Source: CAD feature listing. Evaluate the final solid. Frame: model axes, mm. Face numbers are marked on the shaded views. A direction names the side the tool comes from. Give positions to 0.01 mm unless a question says otherwise; leave off trailing zeros. Order: outer loops, then holes, each group sorted by start corner. A loop starts at its lowest first (then second) coordinate and runs counter-clockwise, first axis right, second up. Notation, with made-up numbers: (83.25, 89) - (93.25, 89) arc R14 cw to (93.25, 102) - close; hole circle Ø11 at (-10.75, -26.5). An arc over 180 degrees is marked (long way). Use CSV: the item, a comma, the result in double quotes.
```python
from build123d import *

# Parameters (mm, degrees)
CUT_EXTRUDE1_DEPTH      = 113.41663578
CUT_EXTRUDE1_DEPTH_BACK = 113.41663578
SKETCH6_R               = 16.9


with BuildPart() as part:
    # Sketch5 → Revolve1 (revolve)
    with BuildSketch(Plane.XY, mode=Mode.PRIVATE) as revolve1_sk:
        with BuildLine():
            Line((25, 0), (42.5, 0))
            Line((42.5, 0), (42.5, 55.2))
            Line((42.5, 55.2), (39.5, 55.2))
            Line((39.5, 55.2), (39.5, 59.5))
            Line((39.5, 59.5), (42.5, 59.5))
            Line((42.5, 59.5), (42.5, 66.8))
            Line((42.5, 66.8), (39.5, 66.8))
            Line((39.5, 66.8), (39.5, 71.1))
            Line((39.5, 71.1), (42.5, 71.1))
            Line((42.5, 71.1), (42.5, 78.4))
            Line((42.5, 78.4), (39.5, 78.4))
            Line((39.5, 78.4), (39.5, 82.7))
            Line((39.5, 82.7), (42.5, 82.7))
            Line((42.5, 82.7), (42.5, 90))
            ThreePointArc((42.5, 90), (21.396553461, 93.745704417), (0, 95))
            Line((0, 95), (0, 90))
            Line((0, 90), (0, 85))
            Line((0, 85), (38, 85))
            Line((38, 85), (38, 49.5))
            Line((38, 49.5), (19, 49.5))
            Line((19, 49.5), (19, 12))
            Line((19, 12), (25, 12))
            Line((25, 12), (25, 0))
        make_face()
    revolve(revolve1_sk.sketch.rotate(Axis((0, 0, 0), (0, 1, 0)), 90), axis=Axis((0, 0, 0), (0, 1, 0)))

    # Sketch6 → Cut-Extrude1 (cut, two sides: drawn at the far end of the back side and taken through both)
    with BuildSketch(Plane.XY.offset(-CUT_EXTRUDE1_DEPTH_BACK)):
        with Locations((0, 27)):
            Circle(SKETCH6_R)
    extrude(amount=CUT_EXTRUDE1_DEPTH + CUT_EXTRUDE1_DEPTH_BACK, mode=Mode.SUBTRACT)


solid = part.part
```
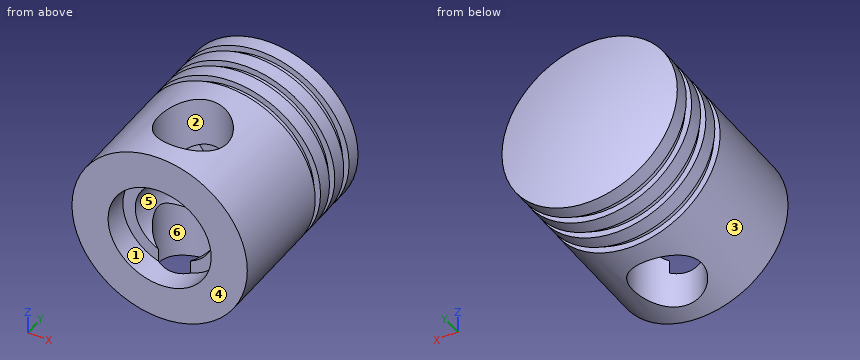
Item 1: Section D-D on y = 73. Return the cut outline in (x, z), then the cut area to 3 significant figures.
Filled in:
outline,"circle Ø85 at (0, 0); hole circle Ø76 at (0, 0)"
area,"1,140 mm2"
Item 2: Material intervals for line 1 (X direction, y = 30, z = 0); line 2 (Y direction, x = 0, z = 31); line 3 (Y direction, x = 6, z = 37), sorted ascending. Write a range as from..to.
Filled in:
line 1,"x = -42.5..-19, 19..42.5"
line 2,"y = 0..10.1, 43.9..49.5, 85..92.36"
line 3,"y = 0..11.2, 42.8..49.5, 85..91.12"
Item 3: First-contact query: pin 1 (5 mm diameter, centred on y = 55, z = 21.5, fed in from +X); pin 2 (14 mm diameter, centred on x = -18.5, z = -9.5, fed in from -Y); pin 3 (6 mm diameter, centred on x = 23, y = 33.5, fed in from +Z); pin 4 (6 mm diameter, centred on y = 58.5, z = 32, fed in from -X). Flat tips, straight axial feed; report the tip coordinate or a pass-through.
Filled in:
pin 1,"stops at x = 38.02"
pin 2,"stops at y = 0"
pin 3,"stops at z = 37.5"
pin 4,"stops at x = -30.91"
Item 4: Section C-C on z = 29.5. Count the separate pieces of the cut face and the enclosed holes in it, then the cut area to 3 significant figures.
Filled in:
separate pieces,"1"
enclosed holes,"2"
area,"2,900 mm2"
Item 5: Section A-A on y = 27. Return the cut outline in (x, z).
Filled in:
outline,"(-16.9, -39) - (-16.9, -8.68) arc R19 cw to (-16.9, 8.68) - (-16.9, 39) arc R42.5 ccw to start; (16.9, -39) arc R42.5 ccw to (16.9, 39) - (16.9, 8.68) arc R19 cw to (16.9, -8.68) - close"
Item 6: Mould query, pull axis X, two halves, no side actions, for the marked faces 3, 4, 5 and 6. Classes: released by +X, released by -X, zero draft, split by the parting line, or undercut.
Filled in:
face 3,"split by the parting line"
face 4,"zero draft"
face 5,"undercut"
face 6,"undercut"
Item 7: Set-up query: the marked faces 1 and 2. Return all of +Z, -Z, +X, -X, +Y, -Y with unobstructed straight access to the full face (end or side cutting, diameter ignored); none if empty.
Filled in:
face 1,"-Y"
face 2,"+Z, -Z"
